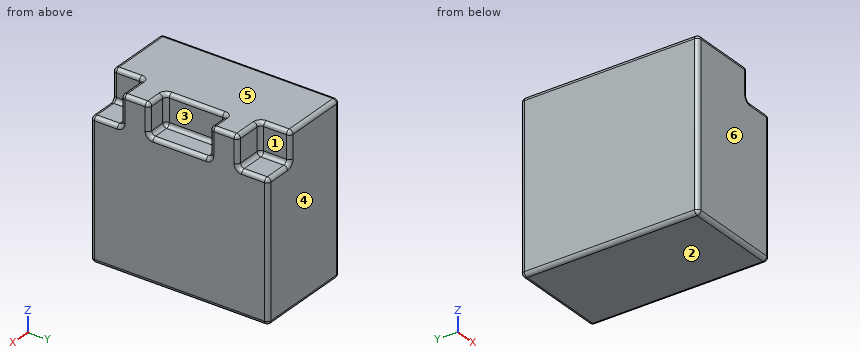
```python
from build123d import *

# Parameters (mm, degrees)
SKETCH1_W           = 82
SKETCH1_H           = 148
BOSS_EXTRUDE1_DEPTH = 140
SKETCH2_W           = 25.4
SKETCH2_H           = 25.4
SKETCH2_W_2         = 19.05
SKETCH2_H_2         = 50.8
CUT_EXTRUDE1_DEPTH  = 25.4
FILLET1_R           = 3.175


with BuildPart() as part:
    # Sketch1 → Boss-Extrude1 (new body)
    with BuildSketch(Plane.XY):
        Rectangle(SKETCH1_W, SKETCH1_H)
    extrude(amount=BOSS_EXTRUDE1_DEPTH)

    # Sketch2 → Cut-Extrude1 (cut)
    with BuildSketch(Plane.XY.offset(140)):
        with Locations((28.3, -61.3)):
            Rectangle(SKETCH2_W, SKETCH2_H)
        with Locations((28.3, 61.3)):
            Rectangle(SKETCH2_W, SKETCH2_H)
        with Locations((31.475, 0)):
            Rectangle(SKETCH2_W_2, SKETCH2_H_2)
    extrude(amount=-CUT_EXTRUDE1_DEPTH, mode=Mode.SUBTRACT)

    # Fillet1
    fillet1_edges = [part.edges().sort_by_distance(p)[0] for p in [
        (41, -37, 140),
        (41, 37, 140),
        (-12.7, 74, 140),
        (41, 74, 57.3),
        (41, -74, 57.3),
        (41, -61.3, 114.6),
        (41, -48.6, 127.3),
        (28.3, -74, 114.6),
        (15.6, -61.3, 114.6),
        (15.6, -74, 127.3),
        (28.3, -48.6, 114.6),
        (15.6, -48.6, 127.3),
        (28.3, -48.6, 140),
        (15.6, -61.3, 140),
        (41, 61.3, 114.6),
        (28.3, 48.6, 114.6),
        (41, 48.6, 127.3),
        (15.6, 61.3, 114.6),
        (15.6, 48.6, 127.3),
        (28.3, 74, 114.6),
        (15.6, 74, 127.3),
        (15.6, 61.3, 140),
        (28.3, 48.6, 140),
        (41, 0, 114.6),
        (41, 25.4, 127.3),
        (31.475, -25.4, 114.6),
        (41, -25.4, 127.3),
        (21.95, 0, 114.6),
        (21.95, -25.4, 127.3),
        (31.475, 25.4, 114.6),
        (21.95, 25.4, 127.3),
        (31.475, 25.4, 140),
        (21.95, 0, 140),
        (31.475, -25.4, 140),
        (-41, 0, 140),
        (0, 74, 0),
        (41, 0, 0),
        (0, -74, 0),
        (-41, 0, 0),
        (-41, 74, 70),
        (-41, -74, 70),
        (-12.7, -74, 140),
    ]]
    fillet(fillet1_edges, radius=FILLET1_R)


solid = part.part
```
Part model, mm, in its own coordinate system. Face numbers are marked on the shaded views. A direction names the side the tool comes from. Round coordinates to 2 decimals unless told otherwise and drop trailing zeros. Loops run counter-clockwise (first coordinate to the right, second up) from the corner with the lowest first, then second, coordinate; pieces in that order, holes last.
Item 1: Mould opens along Y. For the marked faces 3, 4, 5 and 6 say: +Y half, -Y half, draft (parallel to the pull), parting line (faces both ways), or undercut.
Item 2: Cut at B-B, the plane z = 123.5. Give the cut face in (x, y) (3 decimals), then the cut area to 3 significant figures.
Item 3: Cut at C-C, the plane x = 29.5. Give the cut face in (y, z) (3 decimals).
Item 4: Cut at D-D, the plane y = 14.5. Give the cut face in (x, z) (3 decimals), then the cut area to 3 significant figures.
Item 5: Drill centre lines: line 1 (Z direction, x = 27, y = -61); line 2 (Y direction, x = 19, z = 130); line 3 (X direction, y = -28, z = 132). Where is each one in solid material? Low to high.
Item 6: Drop flat-ended pins along their axis: P1, Ø5.5, axis at x = 25.5, y = 65.5, coming from the +Z side; P2, Ø21, axis at x = 31, z = 130, coming from the -Y side; P3, Ø15, axis at y = 64.5, z = 124.5, coming from the +X side. Give the stop position or say it passes through.
Item 7: Cut at A-A, the plane y = -62. Give the cut face in (x, z) (3 decimals).
Item 8: 3-axis set-ups, long thin cutter, end or side, ignore diameter. For the marked faces 1 and 2: which of +Z, -Z, +X, -X, +Y, -Y reach the whole face in a straight line?
A:
1. face 3: undercut
1. face 4: +Y half
1. face 5: draft
1. face 6: -Y half
2. outline: (-41, -70.825) arc R3.175 ccw to (-37.825, -74) - (12.425, -74) arc R3.175 ccw to (15.6, -70.825) - (15.6, -51.775) arc R3.175 cw to (18.775, -48.6) - (37.825, -48.6) arc R3.175 ccw to (41, -45.425) - (41, -28.575) arc R3.175 ccw to (37.825, -25.4) - (25.125, -25.4) arc R3.175 cw to (21.95, -22.225) - (21.95, 22.225) arc R3.175 cw to (25.125, 25.4) - (37.825, 25.4) arc R3.175 ccw to (41, 28.575) - (41, 45.425) arc R3.175 ccw to (37.825, 48.6) - (18.775, 48.6) arc R3.175 cw to (15.6, 51.775) - (15.6, 70.825) arc R3.175 ccw to (12.425, 74) - (-37.825, 74) arc R3.175 ccw to (-41, 70.825) - close
2. area: 9,870 mm2
3. outline: (-74, 3.175) arc R3.175 ccw to (-70.825, 0) - (70.825, 0) arc R3.175 ccw to (74, 3.175) - (74, 111.425) arc R3.175 ccw to (70.825, 114.6) - (51.775, 114.6) arc R3.175 cw to (48.6, 117.775) - (48.6, 136.825) arc R3.175 ccw to (45.425, 140) - (28.575, 140) arc R3.175 ccw to (25.4, 136.825) - (25.4, 117.775) arc R3.175 cw to (22.225, 114.6) - (-22.225, 114.6) arc R3.175 cw to (-25.4, 117.775) - (-25.4, 136.825) arc R3.175 ccw to (-28.575, 140) - (-45.425, 140) arc R3.175 ccw to (-48.6, 136.825) - (-48.6, 117.775) arc R3.175 cw to (-51.775, 114.6) - (-70.825, 114.6) arc R3.175 ccw to (-74, 111.425) - close
4. outline: (-41, 3.175) arc R3.175 ccw to (-37.825, 0) - (37.825, 0) arc R3.175 ccw to (41, 3.175) - (41, 111.425) arc R3.175 ccw to (37.825, 114.6) - (25.125, 114.6) arc R3.175 cw to (21.95, 117.775) - (21.95, 136.825) arc R3.175 ccw to (18.775, 140) - (-37.825, 140) arc R3.175 ccw to (-41, 136.825) - close
4. area: 11,000 mm2
5. line 1: z = 0 to 114.6
5. line 2: y = -48.6 to 48.6
5. line 3: x = -41 to 40.95
6. P1: stops at z = 114.6
6. P2: stops at y = -48.6
6. P3: stops at x = 15.7
7. outline: (-41, 3.175) arc R3.175 ccw to (-37.825, 0) - (37.825, 0) arc R3.175 ccw to (41, 3.175) - (41, 111.425) arc R3.175 ccw to (37.825, 114.6) - (18.775, 114.6) arc R3.175 cw to (15.6, 117.775) - (15.6, 136.825) arc R3.175 ccw to (12.425, 140) - (-37.825, 140) arc R3.175 ccw to (-41, 136.825) - close
8. face 1: +Z, +X, +Y
8. face 2: -Z, +X, -X, +Y, -Y
